Source: CAD feature listing. Evaluate the final solid. Frame: model axes, mm. A direction names the side the tool comes from. Round coordinates to 2 decimals unless told otherwise and drop trailing zeros. Write each loop counter-clockwise with the first axis right and the second up, starting at its lowest first coordinate (ties: lowest second). Pieces come first, ordered by that corner, then holes. Notation, with made-up numbers: (15, 20) - (52, 20) arc R21 cw to (52, 58) - close; hole circle Ø4 at (81, 8.25). An arc over 180 degrees is marked (long way). Write item = value, one per line. Start each with the question number.
```python
from build123d import *

# Parameters (mm, degrees)
SKETCH1_R           = 1.7
BOSS_EXTRUDE1_DEPTH = 3
BOSS_EXTRUDE2_DEPTH = 3
SKETCH3_R           = 3.2
BOSS_EXTRUDE3_DEPTH = 3
SKETCH4_R           = 2.85
SKETCH4_R_2         = 1.7
CUT_EXTRUDE1_DEPTH  = 1.5


with BuildPart() as part:
    # Sketch1 → Boss-Extrude1 (new body)
    with BuildSketch(Plane.XY):
        with BuildLine():
            Line((-56, -43), (56, -43))
            ThreePointArc((56, -43), (58.828427125, -41.828427125), (60, -39))
            Line((60, -39), (60, 39))
            ThreePointArc((60, 39), (58.828427125, 41.828427125), (56, 43))
            Line((56, 43), (-56, 43))
            ThreePointArc((-56, 43), (-58.828427125, 41.828427125), (-60, 39))
            Line((-60, 39), (-60, -39))
            ThreePointArc((-60, -39), (-58.828427125, -41.828427125), (-56, -43))
        make_face()
        with Locations((-54.5, 37.5)):
            Circle(SKETCH1_R, mode=Mode.SUBTRACT)
        with Locations(Location((-54.5, -37.5, 0), (0, 0, 180))):
            Circle(SKETCH1_R, mode=Mode.SUBTRACT)
        with Locations((54.5, -37.5)):
            Circle(SKETCH1_R, mode=Mode.SUBTRACT)
        with Locations(Location((54.5, 37.5, 0), (0, 0, 180))):
            Circle(SKETCH1_R, mode=Mode.SUBTRACT)
    extrude(amount=BOSS_EXTRUDE1_DEPTH)

    # Sketch2 → Boss-Extrude2 (add)
    with BuildSketch(Plane.XY.offset(3)):
        with BuildLine():
            Line((-57.8, 31.601695159), (-57.8, -31.601695159))
            ThreePointArc((-57.8, -31.601695159), (-57.005821231, -33.293932337), (-55.196666667, -33.764406934))
            ThreePointArc((-55.196666667, -33.764406934), (-51.812994231, -34.812994231), (-50.764406934, -38.196666667))
            ThreePointArc((-50.764406934, -38.196666667), (-50.293932337, -40.005821231), (-48.601695159, -40.8))
            Line((-48.601695159, -40.8), (48.601695159, -40.8))
            ThreePointArc((48.601695159, -40.8), (50.293932337, -40.005821231), (50.764406934, -38.196666667))
            ThreePointArc((50.764406934, -38.196666667), (51.812994231, -34.812994231), (55.196666667, -33.764406934))
            ThreePointArc((55.196666667, -33.764406934), (57.005821231, -33.293932337), (57.8, -31.601695159))
            Line((57.8, -31.601695159), (57.8, 31.601695159))
            ThreePointArc((57.8, 31.601695159), (57.005821231, 33.293932337), (55.196666667, 33.764406934))
            ThreePointArc((55.196666667, 33.764406934), (51.812994231, 34.812994231), (50.764406934, 38.196666667))
            ThreePointArc((50.764406934, 38.196666667), (50.293932337, 40.005821231), (48.601695159, 40.8))
            Line((48.601695159, 40.8), (-48.601695159, 40.8))
            ThreePointArc((-48.601695159, 40.8), (-50.293932337, 40.005821231), (-50.764406934, 38.196666667))
            ThreePointArc((-50.764406934, 38.196666667), (-51.812994231, 34.812994231), (-55.196666667, 33.764406934))
            ThreePointArc((-55.196666667, 33.764406934), (-57.005821231, 33.293932337), (-57.8, 31.601695159))
        make_face()
        with BuildLine():
            Line((-48.601695159, 38.8), (48.601695159, 38.8))
            ThreePointArc((48.601695159, 38.8), (48.755534902, 38.72780193), (48.79830532, 38.563333333))
            ThreePointArc((48.79830532, 38.563333333), (50.398780669, 33.398780669), (55.563333333, 31.79830532))
            ThreePointArc((55.563333333, 31.79830532), (55.72780193, 31.755534902), (55.8, 31.601695159))
            Line((55.8, 31.601695159), (55.8, -31.601695159))
            ThreePointArc((55.8, -31.601695159), (55.72780193, -31.755534902), (55.563333333, -31.79830532))
            ThreePointArc((55.563333333, -31.79830532), (50.398780669, -33.398780669), (48.79830532, -38.563333333))
            ThreePointArc((48.79830532, -38.563333333), (48.755534902, -38.72780193), (48.601695159, -38.8))
            Line((48.601695159, -38.8), (-48.601695159, -38.8))
            ThreePointArc((-48.601695159, -38.8), (-48.755534902, -38.72780193), (-48.79830532, -38.563333333))
            ThreePointArc((-48.79830532, -38.563333333), (-50.398780669, -33.398780669), (-55.563333333, -31.79830532))
            ThreePointArc((-55.563333333, -31.79830532), (-55.72780193, -31.755534902), (-55.8, -31.601695159))
            Line((-55.8, -31.601695159), (-55.8, 31.601695159))
            ThreePointArc((-55.8, 31.601695159), (-55.72780193, 31.755534902), (-55.563333333, 31.79830532))
            ThreePointArc((-55.563333333, 31.79830532), (-50.398780669, 33.398780669), (-48.79830532, 38.563333333))
            ThreePointArc((-48.79830532, 38.563333333), (-48.755534902, 38.72780193), (-48.601695159, 38.8))
        make_face(mode=Mode.SUBTRACT)
    extrude(amount=BOSS_EXTRUDE2_DEPTH)

    # Sketch3 → Boss-Extrude3 (add)
    # profile 1 of 2: a face of its own
    with BuildSketch(Plane.XY.offset(3)):
        with BuildLine():
            Line((60, 3), (60, -7))
            Line((60, -7), (60, -27))
            Line((60, -27), (60, -37))
            ThreePointArc((60, -37), (62.928932188, -29.928932188), (70, -27))
            Line((70, -27), (72, -27))
            ThreePointArc((72, -27), (77.656854249, -24.656854249), (80, -19))
            Line((80, -19), (80, -15))
            ThreePointArc((80, -15), (77.656854249, -9.343145751), (72, -7))
            Line((72, -7), (70, -7))
            ThreePointArc((70, -7), (62.928932188, -4.071067812), (60, 3))
        make_face()
        with Locations((70, -17)):
            Circle(SKETCH3_R, mode=Mode.SUBTRACT)
    # profile 2 of 2: a face of its own
    with BuildSketch(Plane.XY.offset(3)):
        with BuildLine():
            Line((-70, -7), (-72, -7))
            ThreePointArc((-72, -7), (-77.656854249, -9.343145751), (-80, -15))
            Line((-80, -15), (-80, -19))
            ThreePointArc((-80, -19), (-77.656854249, -24.656854249), (-72, -27))
            Line((-72, -27), (-70, -27))
            ThreePointArc((-70, -27), (-62.928932188, -29.928932188), (-60, -37))
            Line((-60, -37), (-60, -27))
            Line((-60, -27), (-60, -7))
            Line((-60, -7), (-60, 3))
            ThreePointArc((-60, 3), (-62.928932188, -4.071067812), (-70, -7))
        make_face()
        with Locations(Location((-70, -17, 0), (0, 0, 180))):
            Circle(SKETCH3_R, mode=Mode.SUBTRACT)
    extrude(amount=-BOSS_EXTRUDE3_DEPTH)

    # Sketch4 → Cut-Extrude1 (cut)
    # profile 1 of 4: a face of its own
    with BuildSketch(Plane(origin=(0, 0, 0), x_dir=(-1, 0, 0), z_dir=(0, 0, -1))):
        with Locations((-54.5, 37.5)):
            Circle(SKETCH4_R)
        with Locations((-54.5, 37.5)):
            Circle(SKETCH4_R_2, mode=Mode.SUBTRACT)
    # profile 2 of 4: a face of its own
    with BuildSketch(Plane(origin=(0, 0, 0), x_dir=(-1, 0, 0), z_dir=(0, 0, -1))):
        with Locations((54.5, 37.5)):
            Circle(SKETCH4_R)
        with Locations((54.5, 37.5)):
            Circle(SKETCH4_R_2, mode=Mode.SUBTRACT)
    # profile 3 of 4: a face of its own
    with BuildSketch(Plane(origin=(0, 0, 0), x_dir=(-1, 0, 0), z_dir=(0, 0, -1))):
        with Locations((54.5, -37.5)):
            Circle(SKETCH4_R)
        with Locations((54.5, -37.5)):
            Circle(SKETCH4_R_2, mode=Mode.SUBTRACT)
    # profile 4 of 4: a face of its own
    with BuildSketch(Plane(origin=(0, 0, 0), x_dir=(-1, 0, 0), z_dir=(0, 0, -1))):
        with Locations((-54.5, -37.5)):
            Circle(SKETCH4_R)
        with Locations((-54.5, -37.5)):
            Circle(SKETCH4_R_2, mode=Mode.SUBTRACT)
    extrude(amount=-CUT_EXTRUDE1_DEPTH, mode=Mode.SUBTRACT)


solid = part.part
```
(1) Section A-A (y = 13.5). Return the cut outline in (x, z).
(2) Contact query for flat-ended pins moving along their axis: P1, Ø1, axis at x = -45.5, y = 8, coming from the +Z side; P2, Ø1.7, axis at x = -55.5, y = 37, coming from the -Z side; P3, Ø1, axis at x = -71, z = 1, coming from the -Y side; P4, Ø1.7, axis at x = 54.5, y = -38, coming from the -Z side. Output: stop coordinate, or through.
(3) Pull-direction query (Y, two-part tool) for faces 1 (the flat face through (-1, 1, 0)), 2 (the flat face through (-1, 38.8, 4)), 3 (the cylindrical face through (-63.01, -29.85, 1.52)), 4 (the cylindrical face through (58.859, 41.797, 1.479)); classes: +Y half, -Y half, draft (parallel to the pull), parting line (faces both ways), or undercut.
(4) Ray query, L1, parallel to Y at x = 54.5, z = 0.85; L2, parallel to X at y = -15.5, z = 1.45; L3, parallel to Y at x = -32, z = 3.3. Return the intervals inside material, ascending. Write a range as from..to.
(5) Reachability of faces 5 (the cylindrical face through (53.185, -40.028, 0.74)), 6 (the cylindrical face through (-58.859, -41.797, 1.479)), 7 (the flat face through (55.8, 0, 4)) from +Z, -Z, +X, -X, +Y, -Y: full face, straight path, thin tool, end or side. Return the list, or none.
(6) Section B-B (x = 28). Return the cut outline in (y, z), plus the area to 3 significant figures.
Solution:
q1.outline = (-60, 0) - (60, 0) - (60, 3) - (57.8, 3) - (57.8, 6) - (55.8, 6) - (55.8, 3) - (-55.8, 3) - (-55.8, 6) - (-57.8, 6) - (-57.8, 3) - (-60, 3) - close
q2.P1 = 3
q2.P2 = 1.5
q2.P3 = -27
q2.P4 = through
q3.face_1 = draft
q3.face_2 = undercut
q3.face_3 = -Y half
q3.face_4 = +Y half
q4.L1 = -43..-40.35, -34.65..34.65, 40.35..43
q4.L2 = -80..-72.83, -67.17..67.17, 72.83..80
q4.L3 = -40.8..-38.8, 38.8..40.8
q5.face_5 = -Z
q5.face_6 = +Z, -Z, -X, -Y
q5.face_7 = +Z
q6.outline = (-43, 0) - (43, 0) - (43, 3) - (40.8, 3) - (40.8, 6) - (38.8, 6) - (38.8, 3) - (-38.8, 3) - (-38.8, 6) - (-40.8, 6) - (-40.8, 3) - (-43, 3) - close
q6.area = 270 mm^2
